Design review of the part built by this model. Coordinates are the model's own, in mm. A direction names the side the tool comes from. Give positions to 0.01 mm unless a question says otherwise; leave off trailing zeros. Loops run counter-clockwise (first coordinate to the right, second up) from the corner with the lowest first, then second, coordinate; pieces in that order, holes last. Notation, with made-up numbers: (-37, 7) -> (-8, 7) arc R35 ccw to (-8, 42) -> close; hole circle Ø10 at (45.5, 72.5). An arc over 180 degrees is marked (long way). Answer as CSV lines item,"result".
from build123d import *

# Parameters (mm, degrees)
SKETCH1_W           = 100
SKETCH1_H           = 100
BOSS_EXTRUDE1_DEPTH = 2000
SKETCH2_W           = 40
SKETCH2_H           = 1000
CUT_EXTRUDE1_DEPTH  = 40
SKETCH3_W           = 40
SKETCH3_H           = 1000
CUT_EXTRUDE2_DEPTH  = 40
SKETCH4_W           = 40
SKETCH4_H           = 1750
CUT_EXTRUDE3_DEPTH  = 20
SKETCH5_W           = 40
SKETCH5_H           = 1750
CUT_EXTRUDE4_DEPTH  = 20


with BuildPart() as part:
    # Sketch1 → Boss-Extrude1 (new body)
    with BuildSketch(Plane(origin=(0, 0, 0), x_dir=(1, 0, 0), z_dir=(0, 1, 0))):
        with Locations((6.50810977, -17.305559975)):
            Rectangle(SKETCH1_W, SKETCH1_H)
    extrude(amount=BOSS_EXTRUDE1_DEPTH)

    # Sketch2 → Cut-Extrude1 (cut)
    with BuildSketch(Plane.XY.offset(67.305559975)):
        with Locations((6.50810977, 500)):
            Rectangle(SKETCH2_W, SKETCH2_H)
    extrude(amount=-CUT_EXTRUDE1_DEPTH, mode=Mode.SUBTRACT)

    # Sketch3 → Cut-Extrude2 (cut)
    with BuildSketch(Plane(origin=(0, 0, -32.694440025), x_dir=(-1, 0, 0), z_dir=(0, 0, -1))):
        with Locations((-6.50810977, 1500)):
            Rectangle(SKETCH3_W, SKETCH3_H)
    extrude(amount=-CUT_EXTRUDE2_DEPTH, mode=Mode.SUBTRACT)

    # Sketch4 → Cut-Extrude3 (cut)
    with BuildSketch(Plane(origin=(56.50810977, 0, 0), x_dir=(0, 0, -1), z_dir=(1, 0, 0))):
        with Locations((-17.305559975, 875)):
            Rectangle(SKETCH4_W, SKETCH4_H)
    extrude(amount=-CUT_EXTRUDE3_DEPTH, mode=Mode.SUBTRACT)

    # Sketch5 → Cut-Extrude4 (cut)
    with BuildSketch(Plane.ZY.offset(43.49189023)):
        with Locations((17.305559975, 875)):
            Rectangle(SKETCH5_W, SKETCH5_H)
    extrude(amount=-CUT_EXTRUDE4_DEPTH, mode=Mode.SUBTRACT)


solid = part.part
Q1. For faces 1 (the flat face through (6, 1000, 48)), 2 (the flat face through (-13.492, 1493, -13)), 3 (the flat face through (-23.492, 887, 17)), list the 3-axis set-ups (+Z, -Z, +X, -X, +Y, -Y) from which the entire face can be reached by the end or side of a thin tool; tool diameter is ignored.
Filled sheet:
face 1,"+Z, -Y"
face 2,"-Z, +Y"
face 3,"-X, -Y"
Q2. Clearance check with flat-ended pins moving along their axes: pin 1 Ø20 at (x, z) = (4.5, -12.5) entering from +Y; pin 2 Ø10 at (x, y) = (3.5, 1259.5) entering from -Z; pin 3 Ø6 at (y, z) = (1319, 31) entering from +X. State where each tip first meets the part, or that it passes through.
Filled sheet:
pin 1,"stops at y = 1000"
pin 2,"stops at z = 7.31"
pin 3,"stops at x = 36.51"
Q3. We need section A-A, the plane y = 378.5. State the section outline as (x, z) points, and give its area (3 significant figures).
Filled sheet:
outline,"(-43.49, -32.69) -> (56.51, -32.69) -> (56.51, -2.69) -> (36.51, -2.69) -> (36.51, 37.31) -> (56.51, 37.31) -> (56.51, 67.31) -> (26.51, 67.31) -> (26.51, 27.31) -> (-13.49, 27.31) -> (-13.49, 67.31) -> (-43.49, 67.31) -> (-43.49, 37.31) -> (-23.49, 37.31) -> (-23.49, -2.69) -> (-43.49, -2.69) -> close"
area,"6,800 mm^2"
Q4. To check wall thickness, follow probe 1 along X at (y, z) = (701.5, 30); probe 2 along Z at (x, y) = (46.5, 577); probe 3 along X at (y, z) = (1402.5, -18). State the ranges of each line that lie inside material, in increasing order. Write a range as from..to.
Filled sheet:
probe 1,"x = -23.49..-13.49, 26.51..36.51"
probe 2,"z = -32.69..-2.69, 37.31..67.31"
probe 3,"x = -43.49..-13.49, 26.51..56.51"
Q5. The part is to be moulded in two halves that separate along X. For faces 4 (the flat face through (36.508, 887, 18)), 5 (the flat face through (6, 2000, 17)), 6 (the flat face through (-43.492, 986, -4)), 7 (the flat face through (7, 1507, 7.306)), say which applies: pulls with the +X half, pulls with the -X half, needs draft (parallel to the pull), parting line crosses it, or undercut.
Filled sheet:
face 4,"pulls with the +X half"
face 5,"needs draft"
face 6,"pulls with the -X half"
face 7,"undercut"
